For this review, take the finished solid that the model builds, in its own axes (mm). Coordinates: 2 decimals unless noted, no trailing zeros. Order: outer loops, then holes, each group sorted by start corner. A loop starts at its lowest first (then second) coordinate and runs counter-clockwise, first axis right, second up. Notation, with made-up numbers: M -25,50.25 L -8,50.25 A27 cw -8,88.25 Z; hole C 58,51 d8. An arc over 180 degrees is marked long. Use CSV: the item, a comma, the result in double quotes.
```python
from build123d import *

# Parameters (mm, degrees)
BOSS_EXTRU_1_DEPTH = 150
TROU_TARAUD_M63_D  = 5


with BuildPart() as part:
    # Esquisse1 → Boss.-Extru.1 (new body)
    with BuildSketch(Plane.XY):
        with BuildLine():
            Line((0, 0), (12.5, 0))
            Line((12.5, 0), (6, 13.5))
            ThreePointArc((6, 13.5), (3.310660172, 11.507359313), (0, 12))
            Line((0, 12), (0, 0))
        make_face()
    extrude(amount=BOSS_EXTRU_1_DEPTH)

    # Trou taraudé M63 (through all)
    with Locations(Plane(origin=(0, 6, 25), x_dir=(0, 0, -1), z_dir=(-1, 0, 0))):
        with Locations((0, 0), (-50, 0), (-100, 0)):
            Hole(TROU_TARAUD_M63_D / 2)


solid = part.part
```
Item 1: Add section C-C on x = 3.75. State the section outline as (y, z) points, and give its area (3 significant figures).
Solutions:
outline,"M 0,0 L 11.64,0 L 11.64,150 L 0,150 Z; hole C 6,25 d5; hole C 6,75 d5; hole C 6,125 d5"
area,"1,690 mm^2"
Item 2: To check wall thickness, follow line 1 along Y through (x, z) = (8, 125); line 2 along Y through (x, z) = (3.75, 75); line 3 along X through (y, z) = (7, 107). State the ranges of each line that lie inside material, in increasing order. Write a range as [from, to].
Solutions:
line 1,"[0, 3.5], [8.5, 9.35]"
line 2,"[0, 3.5], [8.5, 11.64]"
line 3,"[0, 9.13]"
Item 3: Clearance check with flat-ended pins moving along their axes: pin 1 Ø2 at (x, y) = (8, 6) entering from -Z; pin 2 Ø4.5 at (y, z) = (6, 75) entering from -X; pin 3 Ø1 at (x, z) = (2, 107.5) entering from +Y; pin 4 Ø2 at (x, z) = (5.5, 86.5) entering from +Y. State where each tip first meets the part, or that it passes through.
Solutions:
pin 1,"z = 0"
pin 2,"through"
pin 3,"y = 11.44"
pin 4,"y = 13.5"
Item 4: Add section A-A on y = 7.25. State the section outline as (x, z) points, and give its area (3 significant figures).
Solutions:
outline,"M 0,0 L 9.01,0 L 9.01,22.83 L 0,22.83 Z; M 0,27.17 L 9.01,27.17 L 9.01,72.83 L 0,72.83 Z; M 0,77.17 L 9.01,77.17 L 9.01,122.83 L 0,122.83 Z; M 0,127.17 L 9.01,127.17 L 9.01,150 L 0,150 Z"
area,"1,230 mm^2"
Item 5: Add section B-B on z = 125. State the section outline as (x, y) points, and give its area (3 significant figures).
Solutions:
outline,"M 0,0 L 12.5,0 L 10.81,3.5 L 0,3.5 Z; M 0,8.5 L 8.41,8.5 L 6,13.5 A4.37 cw 0,12 Z"
area,"66.9 mm^2"
Item 6: Add section D-D on z = 90.5. State the section outline as (x, y) points.
Solutions:
outline,"M 0,0 L 12.5,0 L 6,13.5 A4.37 cw 0,12 Z"
Item 7: Draft analysis for pull direction X (two halves, no side actions). For faces 1 (the face through (7.85, 9.66, 73.95)), 2 (the face through (3.36, 11.52, 73.95)), 3 (the face through (5.5, 3.52, 74.67)), state which applies: released by +X, released by -X, zero draft, split by the parting line, or undercut.
Solutions:
face 1,"released by +X"
face 2,"undercut"
face 3,"zero draft"
